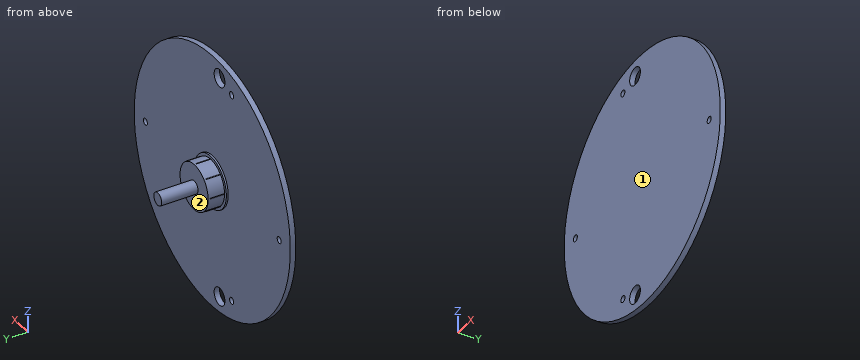
from build123d import *

# Parameters (mm, degrees)
SKETCH1_R                      = 70
BASE_PLATE_DEPTH               = 3
SKETCH2_R                      = 14.25
BEARING_STEPUP_DEPTH           = 1
SKETCH3_R                      = 12.6
BEARING_SITTING_DEPTH          = 9
SKETCH4_R                      = 0.2
BEARING_SITTING_GRID_DEPTH     = 8
SKETCH5_R                      = 1.8
M3_SCREW_CLEARANCE_HOLES_DEPTH = 100.844879688
SKETCH6_R                      = 4.825
HOLES_RESERVED_FOR_RODS_DEPTH  = 100.844879688
SKETCH7_R                      = 3.5
BOSS_EXTRUDE5_DEPTH            = 20


with BuildPart() as part:
    # Sketch1 → base-plate (new body)
    with BuildSketch(Plane(origin=(0, 0, 0), x_dir=(1, 0, 0), z_dir=(0, 1, 0))):
        with Locations(Location((0, 0, 0), (0, 0, 270))):
            Circle(SKETCH1_R)
    extrude(amount=BASE_PLATE_DEPTH)

    # Sketch2 → bearing-stepup (add)
    with BuildSketch(Plane(origin=(0, 3, 0), x_dir=(1, 0, 0), z_dir=(0, 1, 0))):
        with Locations(Location((0, 0, 0), (0, 0, 270))):
            Circle(SKETCH2_R)
    extrude(amount=BEARING_STEPUP_DEPTH)

    # Sketch3 → bearing-sitting (add)
    with BuildSketch(Plane(origin=(0, 4, 0), x_dir=(1, 0, 0), z_dir=(0, 1, 0))):
        with Locations(Location((0, 0, 0), (0, 0, 270))):
            Circle(SKETCH3_R)
    extrude(amount=BEARING_SITTING_DEPTH)

    # Sketch4 → bearing-sitting-grid (add)
    with BuildSketch(Plane(origin=(0, 4, 0), x_dir=(1, 0, 0), z_dir=(0, 1, 0))):
        with Locations((0, 12.6)):
            Circle(SKETCH4_R)
        with Locations((8.909545443, 8.909545443)):
            Circle(SKETCH4_R)
        with Locations((12.6, 0)):
            Circle(SKETCH4_R)
        with Locations((8.909545443, -8.909545443)):
            Circle(SKETCH4_R)
        with Locations((0, -12.6)):
            Circle(SKETCH4_R)
        with Locations((-8.909545443, -8.909545443)):
            Circle(SKETCH4_R)
        with Locations((-12.6, 0)):
            Circle(SKETCH4_R)
        with Locations((-8.909545443, 8.909545443)):
            Circle(SKETCH4_R)
    extrude(amount=BEARING_SITTING_GRID_DEPTH)

    # Sketch5 → m3-screw-clearance-holes (cut, through all)
    with BuildSketch(Plane.XZ):
        with Locations(Location((-17.341907817, 57.439169852, 0), (0, 0, 270))):
            Circle(SKETCH5_R)
        with Locations(Location((-60, 0, 0), (0, 0, 270))):
            Circle(SKETCH5_R)
        with Locations(Location((-17.341907817, -57.439169852, 0), (0, 0, 270))):
            Circle(SKETCH5_R)
        with Locations(Location((60, 0, 0), (0, 0, 270))):
            Circle(SKETCH5_R)
    extrude(amount=-M3_SCREW_CLEARANCE_HOLES_DEPTH, mode=Mode.SUBTRACT)

    # Sketch6 → holes-reserved-for-rods (cut, through all)
    with BuildSketch(Plane.XZ):
        with Locations(Location((-6.5, 61, 0), (0, 0, 270))):
            Circle(SKETCH6_R)
        with Locations(Location((-6.5, -61, 0), (0, 0, 270))):
            Circle(SKETCH6_R)
    extrude(amount=-HOLES_RESERVED_FOR_RODS_DEPTH, mode=Mode.SUBTRACT)

    # Sketch7 → Boss-Extrude5 (add)
    with BuildSketch(Plane(origin=(0, 13, 0), x_dir=(1, 0, 0), z_dir=(0, 1, 0))):
        with Locations(Location((0, 0, 0), (0, 0, 270))):
            Circle(SKETCH7_R)
    extrude(amount=BOSS_EXTRUDE5_DEPTH)


solid = part.part
Source: CAD feature listing. Evaluate the final solid. Frame: model axes, mm. Face numbers are marked on the shaded views. Round coordinates to 2 decimals unless told otherwise and drop trailing zeros. Loops run counter-clockwise (first coordinate to the right, second up) from the corner with the lowest first, then second, coordinate; pieces in that order, holes last. Notation, with made-up numbers: (-13.5, 48) -> (45.5, 48) arc R24 ccw to (45.5, 62) -> close; hole circle Ø3 at (-1, -4.75). An arc over 180 degrees is marked (long way). Answer as a JSON object with one key per item and string values. Group by question number.
Q1. Contact query for flat-ended pins moving along their axis: P1, Ø12, axis at x = 15.5, y = 9.5, coming from the -Z side; P2, Ø4, axis at x = -17.34, z = 57.44, coming from the +Y side. Output: stop coordinate, or through.
Q2. Ray query, line 1 (X direction, y = 0.75, z = 0); line 2 (Z direction, x = -0.5, y = 18); line 3 (Z direction, x = -6, y = 1). Return the intervals inside material, ascending. Write a range as from..to.
Q3. Section query A-A (z = -61). Output: boundary loops of the cut face in (x, y) (3 decimals).
Q4. Section query D-D (z = 41). Output: boundary loops of the cut face in (x, y).
Q5. Mould query, pull axis Y, two halves, no side actions, for the marked faces 1 and 2. Classes: pulls with the +Y half, pulls with the -Y half, needs draft (parallel to the pull), parting line crosses it, or undercut.
Q6. Section query C-C (y = 8). Output: boundary loops of the cut face in (x, z).
Q7. Section query B-B (x = -6.5). Output: boundary loops of the cut face in (y, z) (3 decimals).
Completed:
{
 "1": {"P1": "z = -8.28", "P2": "y = 3"},
 "2": {"line 1": "-70..-61.8, -58.2..58.2, 61.8..70", "line 2": "-3.46..3.46", "line 3": "-69.74..-65.8, -56.2..56.2, 65.8..69.74"},
 "3": {"outline": "(-34.337, 0) -> (-11.325, 0) -> (-11.325, 3) -> (-34.337, 3) -> close; (-1.675, 0) -> (34.337, 0) -> (34.337, 3) -> (-1.675, 3) -> close"},
 "4": {"outline": "(-56.74, 0) -> (56.74, 0) -> (56.74, 3) -> (-56.74, 3) -> close"},
 "5": {"face 1": "pulls with the -Y half", "face 2": "pulls with the +Y half"},
 "6": {"outline": "(-12.6, -0.2) arc R12.6 ccw to (-9.05, -8.77) arc R0.2 ccw (long way) to (-8.77, -9.05) arc R12.6 ccw to (-0.2, -12.6) arc R0.2 ccw (long way) to (0.2, -12.6) arc R12.6 ccw to (8.77, -9.05) arc R0.2 ccw (long way) to (9.05, -8.77) arc R12.6 ccw to (12.6, -0.2) arc R0.2 ccw (long way) to (12.6, 0.2) arc R12.6 ccw to (9.05, 8.77) arc R0.2 ccw (long way) to (8.77, 9.05) arc R12.6 ccw to (0.2, 12.6) arc R0.2 ccw (long way) to (-0.2, 12.6) arc R12.6 ccw to (-8.77, 9.05) arc R0.2 ccw (long way) to (-9.05, 8.77) arc R12.6 ccw to (-12.6, 0.2) arc R0.2 ccw (long way) to start"},
 "7": {"outline": "(0, -69.698) -> (3, -69.698) -> (3, -65.825) -> (0, -65.825) -> close; (0, -56.175) -> (3, -56.175) -> (3, -12.681) -> (4, -12.681) -> (4, -10.794) -> (13, -10.794) -> (13, 10.794) -> (4, 10.794) -> (4, 12.681) -> (3, 12.681) -> (3, 56.175) -> (0, 56.175) -> close; (0, 65.825) -> (3, 65.825) -> (3, 69.698) -> (0, 69.698) -> close"}
}
